Autodesk Inventor part; units mm, degrees
ref_plane "YZ Plane" through (0, 0, 0) normal (1, 0, 0) x (0, 1, 0)
ref_plane "XZ Plane" through (0, 0, 0) normal (0, 1, 0) x (-1, 0, 0)
ref_plane "XY Plane" through (0, 0, 0) normal (0, 0, 1) x (1, 0, 0)
sketch "Sketch1" plane through (0, 0, 0) normal (0, 0, 1) x (1, 0, 0)
  line L0 (0, 4) -> (0, 0) construction
  arc A0 (8.3449, 0.4035) -> (9.5, 6.1037) centre (8.2, 3.4) ccw
  line L1 (0, 0) -> (-21, 0)
  line L2 (-21, 0) -> (-21, 4)
  line L3 (0, 4) -> (0, 0)
  line L4 (-21, 4) -> (0, 4)
  line L5 (0, 4) -> (5, 4)
  line L6 (5, 4) -> (9.5, 6.1037)
  line L7 (0, 0) -> (6, 0)
  line L8 (6, 0) -> (8.6846, 0.4394)
  dimension "d0" = 8.2
  dimension "d1" = 3.4
  dimension "d3" = 6
  dimension "d47" = 21
  dimension "d57" = 4
  dimension "d66" = 5
  dimension "d67" = 9.5
  dimension "d68" = 6
extrude "Extrusion1" add sketch "Sketch1" along normal blind 2.15
sketch "Sketch6" plane through (0, 0, 0) normal (0, 0, -1) x (-1, 0, 0)
  arc A0 (-9.5, 6.1037) -> (-8.6846, 0.4394) centre (-8.2, 3.4) ccw
  point P0 (0, 0)
  point P1 (-3.5529, 0.4208)
  point P2 (-8.8532, 6.2809)
  point P3 (-10.6507, 0.558)
hole "Hole3" at (8.2, 3.4, 0) direction (0, 0, 1) diameter 1.5 depth 1.5 tip angle 118
sketch "Sketch7" plane through (0, 0, 0) normal (0, 0, -1) x (-1, 0, 0)
  circle A0 centre (-8.2, 3.4) radius 0.75
  circle A1 centre (-8.2, 3.4) radius 1.1
  point P0 (0, 0)
  dimension "d44" = 2.2
extrude "Extrusion4" add sketch "Sketch7" along normal blind 0.3
sketch "Sketch8" plane through (0, 0, 2.15) normal (0, 0, 1) x (1, 0, 0)
  arc A0 (8.6846, 0.4394) -> (9.5, 6.1037) centre (8.2, 3.4) ccw
  line L0 (-21, 4) -> (-21, 0)
  line L1 (-21, 4) -> (-21, 0)
  line L2 (-21, 2) -> (-1.49, 2) construction
  line L3 (5, 4) -> (-21, 4)
  line L4 (-21, 0) -> (6, 0)
  line L5 (6, 0) -> (8.6846, 0.4394)
  line L6 (9.5, 6.1037) -> (5, 4)
  point P0 (0, 0)
  point P1 (-14, 2)
  point P2 (-2.5, 2)
  dimension "d48" = 7
  dimension "d49" = 2.5
hole "Hole4" at (-14, 2, 2.15) at (-2.5, 2, 2.15) direction (0, 0, -1) diameter 2.4 end through all
fillet "Fillet3" radius 2 1 edges at (9.5, 6.1037, 1.075)
fillet "Fillet5" radius 2 2 edges at (5, 4, 1.075) (6, 0, 1.075)
fillet "Fillet6" radius 2 1 edges at (-21, 0, 1.075)
properties part number "phalanx_1_tendon_support" material "Aluminum 6061"
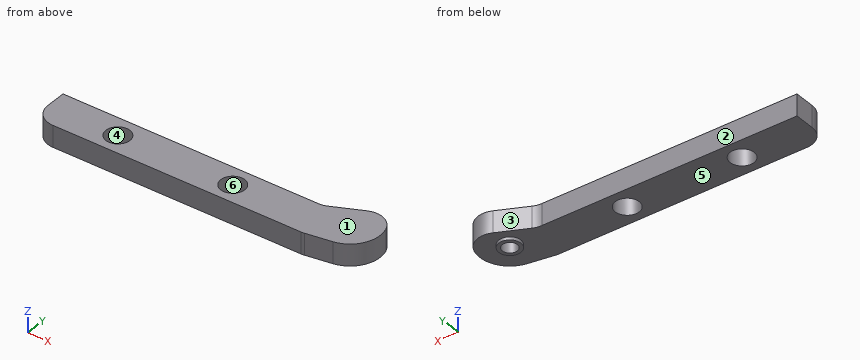
Geometry check sheet. Reference: the model listing, model coordinates, mm. Face numbers are marked on the shaded views. A direction names the side the tool comes from. Coordinates: 2 decimals unless noted, no trailing zeros. Order: outer loops, then holes, each group sorted by start corner. A loop starts at its lowest first (then second) coordinate and runs counter-clockwise, first axis right, second up. Notation, with made-up numbers: (58.5, 1) - (62.5, 1) arc R27 ccw to (62.5, 26) - close; hole circle Ø3 at (81, 64). An arc over 180 degrees is marked (long way). Answer as a JSON object with one key per item and string values. Group by question number.
Item 1: Depth check by flat-ended pin: pin 1 Ø3 at (x, y) = (-2.5, 2) entering from -Z; pin 2 Ø1.1 at (x, z) = (-8.5, 0.5) entering from +Y. Enter the tip coordinate at first touch or a pass-through.
Item 2: Sectioned sample at A-A, the plane z = 0.9. Record the cut outline in (x, y).
Item 3: Draft check along Y on the marked faces 3, 4, 5 and 6. Enter one of: +Y half, -Y half, draft (parallel to the pull), parting line (faces both ways), or undercut.
Item 4: Scan lines: probe 1 along X at (y, z) = (3.4, 1); probe 2 along X at (y, z) = (2, 1.05); probe 3 along Y at (x, z) = (-2.5, 0.5). Record each from-to range of solid material in increasing order.
Item 5: Sectioned sample at B-B, the plane x = -12. Record the cut outline in (y, z).
Item 6: Tool access check on the marked faces 1 and 2. Record the directions out of +Z, -Z, +X, -X, +Y, -Y that give a thin tool (end or side, any length) a straight path to the whole face; none if there is none.
Resolved:
{
 "1": {"pin 1": "z = 0", "pin 2": "y = 4"},
 "2": {"outline": "(-21, 2) arc R2 ccw to (-19, 0) - (5.84, 0) arc R2 ccw to (6.16, 0.03) - (8.68, 0.44) arc R3 ccw to (11.03, 4.39) arc R2 ccw to (8.3, 5.54) - (5.4, 4.19) arc R2 cw to (4.56, 4) - (-21, 4) - close; hole circle Ø2.4 at (-14, 2); hole circle Ø2.4 at (-2.5, 2); hole circle Ø1.5 at (8.2, 3.4)"},
 "3": {"face 3": "+Y half", "face 4": "undercut", "face 5": "draft", "face 6": "undercut"},
 "4": {"probe 1": "-21 to 7.45, 8.95 to 11.2", "probe 2": "-21 to -15.2, -12.8 to -3.7, -1.3 to 10.85", "probe 3": "0 to 0.8, 3.2 to 4"},
 "5": {"outline": "(0, 0) - (4, 0) - (4, 2.15) - (0, 2.15) - close"},
 "6": {"face 1": "+Z, +X, -X, +Y, -Y", "face 2": "+Z, -Z, -X, +Y"}
}
